from build123d import *

# Parameters (mm, degrees)
F2_R     = 19.05
F3_DEPTH = 76.2
F4_R     = 34.925
F5_DEPTH = 76.2


with BuildPart() as f1:
    # F0 (on Front) → F1 (revolve)
    with BuildSketch(Plane.XZ):
        Polygon((0, 180.086), (0, 0), (76.2, 0), (76.2, 12.7), (57.15, 12.7), (57.15, 167.386), (76.2, 167.386), (76.2, 180.086), align=None)
        Polygon((76.2, 0), (0, 0), (0, -50.8), (57.15, -50.8), (57.15, -12.7), (76.2, -12.7), align=None)
        Polygon((0, 230.886), (0, 180.086), (76.2, 180.086), (76.2, 192.786), (57.15, 192.786), (57.15, 230.886), align=None)
    revolve(axis=Axis((0, 0, 90.043), (0, 0, 1)))

    # F2 (on face) → F3 (cut)
    with BuildSketch(Plane(origin=(0, 0, -50.8), x_dir=(1, 0, 0), z_dir=(0, 0, -1))):
        Circle(F2_R)
    extrude(amount=-F3_DEPTH, mode=Mode.SUBTRACT)

    # F4 (on face) → F5 (cut)
    with BuildSketch(Plane.XY.offset(230.886)):
        Circle(F4_R)
    extrude(amount=-F5_DEPTH, mode=Mode.SUBTRACT)


solid = f1.part
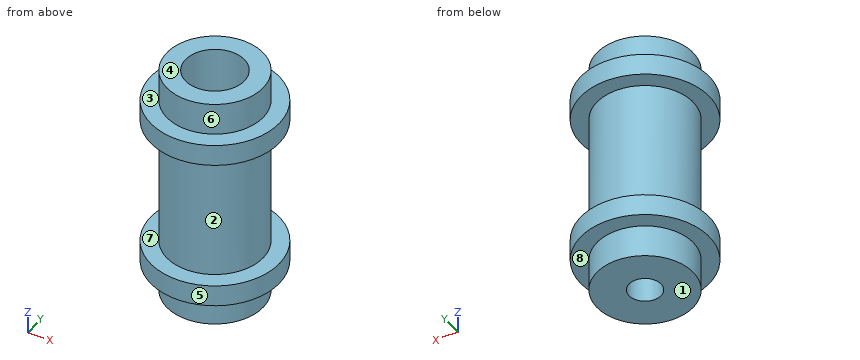
For this review, take the finished solid that the model builds, in its own axes (mm). Face numbers are marked on the shaded views. A direction names the side the tool comes from. Give positions to 0.01 mm unless a question says otherwise; leave off trailing zeros. Loops run counter-clockwise (first coordinate to the right, second up) from the corner with the lowest first, then second, coordinate; pieces in that order, holes last.
Item 1: For line 1 along Y through (x, z) = (0, 172.5) (3 decimals); line 2 along Y through (x, z) = (0, 193.5) (3 decimals); line 3 along Z through (x, y) = (23.5, -64), list the stretches that pass through material, from the lowest coordinate up.
Item 2: Take a section at A-A, the plane x = 0. State the section outline as (y, z) points (3 decimals).
Item 3: Take a section at C-C, the plane z = 50.5. State the section outline as (x, y) points.
Item 4: Tool access review of the marked faces 4, 5, 6, 7 and 8: name each direction out of +Z, -Z, +X, -X, +Y, -Y from which nothing blocks a thin tool from reaching the whole face with its end or side.
Item 5: Take a section at D-D, the plane x = -45. State the section outline as (y, z) points.
Item 6: Draft analysis for pull direction Z (two halves, no side actions). For the marked faces 1, 2 and 3, state which applies: +Z half, -Z half, draft (parallel to the pull), parting line (faces both ways), or undercut.
Item 7: Insertion check: pin 1 (10 mm diameter, centred on x = 39.5, z = 155, fed in from +Y); pin 2 (8 mm diameter, centred on x = -43, y = 46.5, fed in from -Z); pin 3 (2 mm diameter, centred on x = -60, y = 16, fed in from +Z). Each pin has a flat end and moves straight along its axis. Give the tip position at first contact, or say it passes through.
Calculated:
1. line 1: y = -76.2 to -34.925, 34.925 to 76.2
1. line 2: y = -57.15 to -34.925, 34.925 to 57.15
1. line 3: z = -12.7 to 12.7, 167.39 to 192.79
2. outline: (-76.2, -12.7) - (-57.15, -12.7) - (-57.15, -50.8) - (-19.05, -50.8) - (-19.05, 25.4) - (19.05, 25.4) - (19.05, -50.8) - (57.15, -50.8) - (57.15, -12.7) - (76.2, -12.7) - (76.2, 12.7) - (57.15, 12.7) - (57.15, 167.386) - (76.2, 167.386) - (76.2, 192.786) - (57.15, 192.786) - (57.15, 230.886) - (34.925, 230.886) - (34.925, 154.686) - (-34.925, 154.686) - (-34.925, 230.886) - (-57.15, 230.886) - (-57.15, 192.786) - (-76.2, 192.786) - (-76.2, 167.386) - (-57.15, 167.386) - (-57.15, 12.7) - (-76.2, 12.7) - close
3. outline: circle Ø114.3 at (0, 0)
4. face 4: +Z, +X, -X, +Y, -Y
4. face 5: +Z, -Z
4. face 6: +Z
4. face 7: none
4. face 8: -Z
5. outline: (-61.49, -12.7) - (-35.23, -12.7) - (-35.23, -50.8) - (35.23, -50.8) - (35.23, -12.7) - (61.49, -12.7) - (61.49, 12.7) - (35.23, 12.7) - (35.23, 167.39) - (61.49, 167.39) - (61.49, 192.79) - (35.23, 192.79) - (35.23, 230.89) - (-35.23, 230.89) - (-35.23, 192.79) - (-61.49, 192.79) - (-61.49, 167.39) - (-35.23, 167.39) - (-35.23, 12.7) - (-61.49, 12.7) - close
6. face 1: -Z half
6. face 2: undercut
6. face 3: +Z half
7. pin 1: stops at y = 45.56
7. pin 2: stops at z = -12.7
7. pin 3: stops at z = 192.79
